Geometry: final body of the model. Coordinates: model frame, mm. A direction names the side the tool comes from. Coordinates: 2 decimals unless noted, no trailing zeros. Loops run counter-clockwise (first coordinate to the right, second up) from the corner with the lowest first, then second, coordinate; pieces in that order, holes last. Notation, with made-up numbers: (24.5, -26.5) - (30.5, -26.5) arc R7 ccw to (30.5, -18.5) - close; hole circle Ø9 at (72, -18.75). An arc over 180 degrees is marked (long way). Return JSON: item names as keys, results as strings.
Autodesk Inventor part; units mm, degrees
ref_plane "YZ Plane" through (0, 0, 0) normal (1, 0, 0) x (0, 1, 0)
ref_plane "XZ Plane" through (0, 0, 0) normal (0, 1, 0) x (-1, 0, 0)
ref_plane "XY Plane" through (0, 0, 0) normal (0, 0, 1) x (1, 0, 0)
sketch "Эскиз1" plane through (0, 0, 0) normal (0, 0, 1) x (1, 0, 0)
  line L0 (0, 0) -> (0, 20)
  line L1 (0, 20) -> (2.8284, 22.8284)
  line L2 (0, 0) -> (15, 0)
  line L3 (15, 0) -> (15, 20)
  line L4 (15, 20) -> (12.1716, 22.8284)
  line L5 (2.8284, 22.8284) -> (12.1716, 22.8284)
  dimension "d0" = 20
  dimension "d1" = 4
  dimension "d2" = 135
  dimension "d3" = 15
  dimension "d4" = 4
  dimension "d5" = 135
revolve "Вращение1" add sketch "Эскиз1" angle 360 about axis through (0, 0, 0) along (1, 0, 0)
sketch "Эскиз2" plane through (0, 0, 0) normal (-1, 0, 0) x (0, 0, 1)
  point P0 (0, 0)
  point P1 (0, 18)
  point P2 (-15.5885, 9)
  point P3 (-15.5885, -9)
  point P4 (0, -18)
  point P5 (15.5885, -9)
  point P6 (15.5885, 9)
  dimension "d7" = 18
  dimension "d10" = 360
hole "Отверстие1" at (0, 18, 0) at (0, 9, -15.5885) at (0, -9, -15.5885) at (0, -18, 0) at (0, -9, 15.5885) at (0, 9, 15.5885) direction (1, 0, 0) diameter 4 depth 4
sketch "Эскиз3" plane through (0, 0, 0) normal (0, 0, 1) x (1, 0, 0)
  line L0 (0, 0) -> (0, 11)
  line L1 (0, 11) -> (3, 8)
  line L2 (3, 8) -> (8, 8)
  line L3 (8, 8) -> (8, 10.5)
  line L4 (8, 10.5) -> (9, 9.5)
  line L5 (9, 9.5) -> (14, 9.5)
  line L6 (14, 9.5) -> (15, 10.5)
  line L7 (15, 10.5) -> (15, 0)
  line L8 (15, -20) -> (15, 20)
  line L9 (0, 0) -> (15, 0)
  dimension "d19" = 45
  dimension "d20" = 45
  dimension "d21" = 45
  dimension "d22" = 16
  dimension "d23" = 19
  dimension "d24" = 5
  dimension "d25" = 5
  dimension "d26" = 10.5
revolve "Вращение2" cut sketch "Эскиз3" angle 360 about axis through (0, 0, 0) along (1, 0, 0)
properties part number "711135"
Item 1: Section query A-A, the plane x = 2. Return loops of the section in (y, z), and give its area (3 significant figures).
Worked out:
{"outline": "circle Ø44 at (0, 0); hole circle Ø4 at (-18, 0); hole circle Ø4 at (-9, -15.59); hole circle Ø4 at (-9, 15.59); hole circle Ø18 at (0, 0); hole circle Ø4 at (9, -15.59); hole circle Ø4 at (9, 15.59); hole circle Ø4 at (18, 0)", "area": "1,190 mm^2"}
Item 2: Reachability of faces 5 (the face through (8, -2, -8)), 6 (the face through (4, 9, 16)), 7 (the face through (11.54, 4.38, -8.43)) from +Z, -Z, +X, -X, +Y, -Y: full face, straight path, thin tool, end or side. Return the list, or none.
Worked out:
{"face 5": "none", "face 6": "-X", "face 7": "+X"}
Item 3: First-contact query: pin 1 Ø1.2 at (y, z) = (-17.5, 0) entering from -X; pin 2 Ø2 at (x, y) = (11.5, -11.5) entering from +Z; pin 3 Ø8 at (x, z) = (7.5, -4.5) entering from -Y. Flat tips, straight axial feed; report the tip coordinate or a pass-through.
Worked out:
{"pin 1": "x = 4", "pin 2": "z = 20.27", "pin 3": "y = -22.82"}
Item 4: Ray query, probe 1 along Y at (x, z) = (11.5, -0.5); probe 2 along Y at (x, z) = (1.8, 0); probe 3 along Z at (x, y) = (2.75, -9.5) (3 decimals). Return the intervals inside material, ascending. Write a range as from..to.
Worked out:
{"probe 1": "-22.82..-9.49, 9.49..22.82", "probe 2": "-21.8..-20, -16..-9.2, 9.2..16, 20..21.8", "probe 3": "-20.672..-17.525, -13.652..13.652, 17.525..20.672"}
Item 5: Section query B-B, the plane x = 6.25. Return loops of the section in (y, z), and give its area (3 significant figures).
Worked out:
{"outline": "circle Ø45.66 at (0, 0); hole circle Ø16 at (0, 0)", "area": "1,440 mm^2"}
Item 6: Mould query, pull axis Z, two halves, no side actions, for faces 1 (the face through (0, 9, -9)), 2 (the face through (7.565, -4.949, -22.286)), 3 (the face through (4, 18, 0)), 4 (the face through (4, -9, -16)). Classes: +Z half, -Z half, draft (parallel to the pull), parting line (faces both ways), or undercut.
Worked out:
{"face 1": "draft", "face 2": "parting line", "face 3": "undercut", "face 4": "undercut"}
